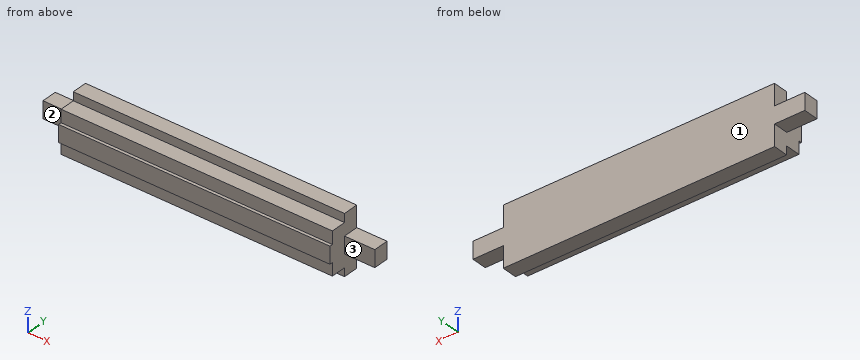
from build123d import *

# Parameters (mm, degrees)
F0_W     = 448
F0_H     = 14
F0_H_2   = 21
F0_W_2   = 50
F0_H_3   = 28
F1_DEPTH = 25
F2_W     = 448
F2_H     = 21
F3_DEPTH = 25
F4_W     = 448
F4_H     = 28
F5_DEPTH = 30


with BuildPart() as f1:
    # F0 (on Front) → F1 (new body)
    with BuildSketch(Plane.XZ):
        with Locations((0, -42)):
            Rectangle(F0_W, F0_H)
        with Locations((0, -24.5)):
            Rectangle(F0_W, F0_H_2)
        with Locations((249, 0)):
            Rectangle(F0_W_2, F0_H_3)
        Rectangle(F0_W, F0_H_3)
        with Locations((-249, 0)):
            Rectangle(F0_W_2, F0_H_3)
        with Locations((0, 24.5)):
            Rectangle(F0_W, F0_H_2)
        with Locations((0, 42)):
            Rectangle(F0_W, F0_H)
    extrude(amount=F1_DEPTH)

    # F2 (on face) → F3 (join)
    with BuildSketch(Plane.XZ.offset(25)):
        with Locations((0, 24.5)):
            Rectangle(F2_W, F2_H)
        with Locations((0, -24.5)):
            Rectangle(F2_W, F2_H)
    extrude(amount=F3_DEPTH)

    # F4 (on face) → F5 (join)
    with BuildSketch(Plane.XZ.offset(25)):
        Rectangle(F4_W, F4_H)
    extrude(amount=F5_DEPTH)


solid = f1.part
Part model, mm, in its own coordinate system. Face numbers are marked on the shaded views. A direction names the side the tool comes from. Give positions to 0.01 mm unless a question says otherwise; leave off trailing zeros. Loops run counter-clockwise (first coordinate to the right, second up) from the corner with the lowest first, then second, coordinate; pieces in that order, holes last. Notation, with made-up numbers: (13, 34.5) -> (21, 34.5) arc R19 ccw to (21, 49.5) -> close; hole circle Ø4 at (-34, 51.25). An arc over 180 degrees is marked (long way). Write each question's results on one line, items separated by ' | '. Start each with the question number.
Q1. Band-saw the part on C-C on z = 3. List the corners of the cut face in (x, y), plus the area to 3 significant figures.
Q2. Band-saw the part on D-D on y = -35.5. List the corners of the cut face in (x, z), plus the area to 3 significant figures.
Q3. Pin check, flat tips, straight feed: P1, Ø12.5, axis at x = 86, y = -34, coming from the -Z side; P2, Ø7.5, axis at x = -237.5, y = -11, coming from the -Z side; P3, Ø5, axis at x = 58, y = -40, coming from the +Z side. Stop position of each tip, or through.
Q4. Band-saw the part on A-A on x = 152. List the corners of the cut face in (y, z), plus the area to 3 significant figures.
Q5. Wall check: L1, parallel to Y at x = -147, z = 32.5; L2, parallel to Z at x = -240.5, y = -17.5; L3, parallel to X at y = -7.5, z = -34.5. Give the ranges that are in metal, low to high.
Q6. Band-saw the part on B-B on y = -15. List the corners of the cut face in (x, z).
Q7. Which spindle directions (+Z, -Z, +X, -X, +Y, -Y) get a long thin tool onto all of the face, cutting with end or side? Do the marked faces 1, 2 and 3. Say none if no direction does.
Results are:
1) outline: (-274, -25) -> (-224, -25) -> (-224, -55) -> (224, -55) -> (224, -25) -> (274, -25) -> (274, 0) -> (-274, 0) -> close | area: 27,100 mm²
2) outline: (-224, -35) -> (224, -35) -> (224, 35) -> (-224, 35) -> close | area: 31,400 mm²
3) P1: stops at z = -35 | P2: stops at z = -14 | P3: stops at z = 35
4) outline: (-55, -14) -> (-50, -14) -> (-50, -35) -> (-25, -35) -> (-25, -49) -> (0, -49) -> (0, 49) -> (-25, 49) -> (-25, 35) -> (-50, 35) -> (-50, 14) -> (-55, 14) -> close | area: 4,340 mm²
5) L1: y = -50 to 0 | L2: z = -14 to 14 | L3: x = -224 to 224
6) outline: (-274, -14) -> (-224, -14) -> (-224, -49) -> (224, -49) -> (224, -14) -> (274, -14) -> (274, 14) -> (224, 14) -> (224, 49) -> (-224, 49) -> (-224, 14) -> (-274, 14) -> close
7) face 1: +Z, -Z, +X, -X, +Y | face 2: +Z, -Z, -X, -Y | face 3: +Z, -Z, +X, -Y
